Design review of the part built by this model. Coordinates are the model's own, in mm. A direction names the side the tool comes from. Give positions to 0.01 mm unless a question says otherwise; leave off trailing zeros. Write each loop counter-clockwise with the first axis right and the second up, starting at its lowest first coordinate (ties: lowest second). Pieces come first, ordered by that corner, then holes.
```python
from build123d import *

# Parameters (mm, degrees)
SKETCH_2_R          = 3.25
CUT_EXTRUDE_1_DEPTH = 3.1
SKETCH_3_R          = 1.75
CUT_EXTRUDE_2_DEPTH = 40.855990767


with BuildPart() as part:
    # 草图1 → 旋转1 (revolve)
    with BuildSketch(Plane.XY):
        Polygon((-17.5, 13.5), (-17.5, 11), (-10.5, 11), (-10.5, 9), (10.5, 9), (10.5, 11), (17.5, 11), (17.5, 13.5), (-4.5, 13.5), (-4.5, 23.5), (-12.5, 23.5), (-12.5, 13.5), align=None)
    revolve(axis=Axis((0, 0, 0), (-1, 0, 0)))

    # 草图2 → 切除-拉伸1 (cut)
    with BuildSketch(Plane(origin=(-4.5, 0, 0), x_dir=(0, 0, -1), z_dir=(1, 0, 0))):
        with Locations(Location((0, 18.5, 0), (0, 0, 90))):
            Circle(SKETCH_2_R)
        with Locations(Location((0, -18.5, 0), (0, 0, 90))):
            Circle(SKETCH_2_R)
        with Locations(Location((18.5, 0, 0), (0, 0, 90))):
            Circle(SKETCH_2_R)
        with Locations(Location((-18.5, 0, 0), (0, 0, 90))):
            Circle(SKETCH_2_R)
    extrude(amount=-CUT_EXTRUDE_1_DEPTH, mode=Mode.SUBTRACT)

    # 草图3 → 切除-拉伸2 (cut, through all)
    with BuildSketch(Plane(origin=(-4.5, 0, 0), x_dir=(0, 0, -1), z_dir=(1, 0, 0))):
        with Locations(Location((0, 18.5, 0), (0, 0, 90))):
            Circle(SKETCH_3_R)
        with Locations(Location((18.5, 0, 0), (0, 0, 90))):
            Circle(SKETCH_3_R)
        with Locations(Location((0, -18.5, 0), (0, 0, 270))):
            Circle(SKETCH_3_R)
        with Locations(Location((-18.5, 0, 0), (0, 0, 90))):
            Circle(SKETCH_3_R)
    extrude(amount=-CUT_EXTRUDE_2_DEPTH, mode=Mode.SUBTRACT)


solid = part.part
```
(1) Consider section D-D, the plane x = 13.5. Give the boundary of the cut face in (y, z), then the cut area to 3 significant figures.
Resolved:
outline: circle Ø27 at (0, 0); hole circle Ø22 at (0, 0)
area: 192 mm2
(2) To check wall thickness, follow L1, parallel to X at y = -17, z = 10.5; L2, parallel to Y at x = 4, z = 0; L3, parallel to Z at x = 12.25, y = 0. State the ranges of each line that lie inside material, in increasing order.
Resolved:
L1: x = -12.5 to -4.5
L2: y = -13.5 to -9, 9 to 13.5
L3: z = -13.5 to -11, 11 to 13.5
(3) Mouldability with a two-part tool opening along Z and no side actions: class faces 4 (the face through (-8.6, 22.4, -7.1)), 5 (the face through (-17.5, -5, 10)), 6 (the face through (-10.02, 16.75, 0.08)) as pulls with the +Z half, pulls with the -Z half, needs draft (parallel to the pull), parting line crosses it, or undercut.
Resolved:
face 4: parting line crosses it
face 5: needs draft
face 6: undercut
(4) Consider section A-A, the plane z = -18.5. Give the boundary of the cut face in (x, y), then the cut area to 3 significant figures.
Resolved:
outline: (-12.5, -14.49) - (-4.5, -14.49) - (-4.5, -3.25) - (-7.6, -3.25) - (-7.6, -1.75) - (-12.5, -1.75) - close; (-12.5, 1.75) - (-7.6, 1.75) - (-7.6, 3.25) - (-4.5, 3.25) - (-4.5, 14.49) - (-12.5, 14.49) - close
area: 195 mm2
(5) Consider section B-B, the plane x = -11.5. Give the boundary of the cut face in (y, z).
Resolved:
outline: circle Ø47 at (0, 0); hole circle Ø3.5 at (-18.5, 0); hole circle Ø22 at (0, 0); hole circle Ø3.5 at (0, -18.5); hole circle Ø3.5 at (0, 18.5); hole circle Ø3.5 at (18.5, 0)
(6) Tool access review of faces 1 (the face through (-12.5, 10, 10)), 2 (the face through (-6.028, -0.423, 21.722)), 3 (the face through (-10.02, -16.75, -0.08)): name each direction out of +Z, -Z, +X, -X, +Y, -Y from which nothing blocks a thin tool from reaching the whole face with its end or side.
Resolved:
face 1: -X
face 2: +X
face 3: +X, -X
(7) Consider section C-C, the plane y = 5.5. Give the boundary of the cut face in (x, z), then the cut area to 3 significant figures.
Resolved:
outline: (-17.5, -12.33) - (-12.5, -12.33) - (-12.5, -22.85) - (-4.5, -22.85) - (-4.5, -12.33) - (17.5, -12.33) - (17.5, -9.53) - (10.5, -9.53) - (10.5, -7.12) - (-10.5, -7.12) - (-10.5, -9.53) - (-17.5, -9.53) - close; (-17.5, 9.53) - (-10.5, 9.53) - (-10.5, 7.12) - (10.5, 7.12) - (10.5, 9.53) - (17.5, 9.53) - (17.5, 12.33) - (-4.5, 12.33) - (-4.5, 22.85) - (-12.5, 22.85) - (-12.5, 12.33) - (-17.5, 12.33) - close
area: 465 mm2
(8) Clearance check with flat-ended pins moving along their axes: P1, Ø2, axis at y = -1, z = 17.5, coming from the +X side; P2, Ø4, axis at y = -18.5, z = 0, coming from the -X side; P3, Ø6, axis at x = -6, z = 8.5, coming from the +Y side. State where each tip first meets the part, or that it passes through.
Resolved:
P1: stops at x = -7.6
P2: stops at x = -12.5
P3: stops at y = 22.85
